The model under review builds one solid part; all positions refer to its coordinate system, in mm. A direction names the side the tool comes from. Coordinates: 2 decimals unless noted, no trailing zeros. Put each result on its own line as item: value.
from build123d import *

# Parameters (mm, degrees)
SHELL2_T           = -4
CUT_EXTRUDE1_DEPTH = 3.175
SKETCH6_W          = 2.767139064
SKETCH6_H          = 25
CUT_EXTRUDE2_DEPTH = 10


with BuildPart() as part:
    # Sketch2 → Loft2 section 0
    with BuildSketch(Plane(origin=(0, 60, 0), x_dir=(1, 0, 0), z_dir=(0, 1, 0))):
        with BuildLine():
            Line((-150, -24.473684211), (-150, 90))
            Line((-150, 90), (150, 90))
            Line((150, 90), (150, -24.473684211))
            Line((150, -24.473684211), (30, -75))
            Line((30, -75), (-30, -75))
            Line((-30, -75), (-150, -24.473684211))
        make_face()
    # Sketch1 → Loft2 section 1
    with BuildSketch(Plane(origin=(0, 0, 0), x_dir=(1, 0, 0), z_dir=(0, 1, 0))):
        with BuildLine():
            Line((125, -35), (125, 35))
            Line((125, 35), (-125, 35))
            Line((-125, 35), (-125, -35))
            Line((-125, -35), (-30, -75))
            Line((-30, -75), (30, -75))
            Line((30, -75), (125, -35))
        make_face()
    loft()

    # Shell2
    shell2_openings = [part.faces().sort_by_distance(p)[0] for p in [
        (0, 60, -16.664896975),
        (0, 30, 75),
    ]]
    offset(amount=SHELL2_T, openings=shell2_openings, kind=Kind.INTERSECTION)

    # Sketch5 → Cut-Extrude1 (cut)
    with BuildSketch(Plane.XY.offset(75)):
        Polygon((-26.825, 3.175), (-15, 3.175), (-15, 0), (15, 0), (15, 3.175), (26.825, 3.175), (26.825, 15.675), (30, 15.675), (30, 40.675), (26.825, 40.675), (26.825, 60), (-26.825, 60), (-26.825, 40.675), (-30, 40.675), (-30, 15.675), (-26.825, 15.675), align=None)
    extrude(amount=-CUT_EXTRUDE1_DEPTH, mode=Mode.SUBTRACT)

    # Sketch6 → Cut-Extrude2 (cut)
    with BuildSketch(Plane.XY.offset(71.825)):
        with Locations((-28.616430468, 28.175)):
            Rectangle(SKETCH6_W, SKETCH6_H)
        with Locations((28.616430468, 28.175)):
            Rectangle(SKETCH6_W, SKETCH6_H)
    extrude(amount=-CUT_EXTRUDE2_DEPTH, mode=Mode.SUBTRACT)


solid = part.part
1. Machinability: for faces 1 (the flat face through (-4, 4, 6)), 2 (the flat face through (28, 4, 75)), which of the approach directions +Z, -Z, +X, -X, +Y, -Y give a long, thin tool a straight path to every point of the face, cutting with its end or side? Answer none if there is none.
Determined:
face 1: +Y
face 2: +Z, +X, -X, +Y, -Y
2. For pin 1 Ø5 at (y, z) = (31, -3.5) entering from -X; pin 2 Ø2.5 at (x, z) = (-18.5, 73) entering from +Y; pin 3 Ø3.5 at (y, z) = (30.5, 72.5) entering from -X, all flat-tipped, find the tip position at first contact; note any pin that passes through.
Determined:
pin 1: stops at x = -138.96
pin 2: stops at y = 4
pin 3: stops at x = -40.09
3. The part is to be moulded in two halves that separate along X. For faces 3 (the flat face through (-27, 4, 75)), 4 (the flat face through (134.569, 33.365, -11.637)), say which applies: +X half, -X half, draft (parallel to the pull), parting line (faces both ways), or undercut.
Determined:
face 3: draft
face 4: undercut
4. To check wall thickness, follow probe 1 along Z at (x, y) = (104.5, 56.5); probe 2 along Z at (x, y) = (-92.5, 54); probe 3 along Y at (x, z) = (11.5, -31.5). State the ranges of each line that lie inside material, in increasing order.
Determined:
probe 1: z = -86.79 to -81.37, 39.29 to 43.63
probe 2: z = -84.5 to -79.07, 44.34 to 48.68
probe 3: y = 0 to 4
